For this review, take the finished solid that the model builds, in its own axes (mm). Face numbers are marked on the shaded views. Give positions to 0.01 mm unless a question says otherwise; leave off trailing zeros. Loops run counter-clockwise (first coordinate to the right, second up) from the corner with the lowest first, then second, coordinate; pieces in that order, holes last. Notation, with made-up numbers: (26, -25) - (74, -25) arc R16 ccw to (74, -14) - close; hole circle Ø8 at (-28.5, 68.5). An arc over 180 degrees is marked (long way). Answer in a Markdown table with one row per item.
```python
from build123d import *

# Parameters (mm, degrees)
ESQUISSE1_R        = 77.9
ESQUISSE1_R_2      = 2.25
ESQUISSE1_R_3      = 5
BOSS_EXTRU_1_DEPTH = 2


with BuildPart() as part:
    # Esquisse1 → Boss.-Extru.1 (new body)
    with BuildSketch(Plane.XY):
        with Locations((0.071120791, 0.517607885)):
            Circle(ESQUISSE1_R)
        with Locations((0.071120791, 73.017607885)):
            Circle(ESQUISSE1_R_2, mode=Mode.SUBTRACT)
        with Locations((72.571120791, 0.517607885)):
            Circle(ESQUISSE1_R_2, mode=Mode.SUBTRACT)
        with Locations((0.071120791, -71.982392115)):
            Circle(ESQUISSE1_R_2, mode=Mode.SUBTRACT)
        with Locations((-72.428879209, 0.517607885)):
            Circle(ESQUISSE1_R_2, mode=Mode.SUBTRACT)
        with Locations((0.071120791, 0.517607885)):
            Circle(ESQUISSE1_R_3, mode=Mode.SUBTRACT)
    extrude(amount=BOSS_EXTRU_1_DEPTH)


solid = part.part
```
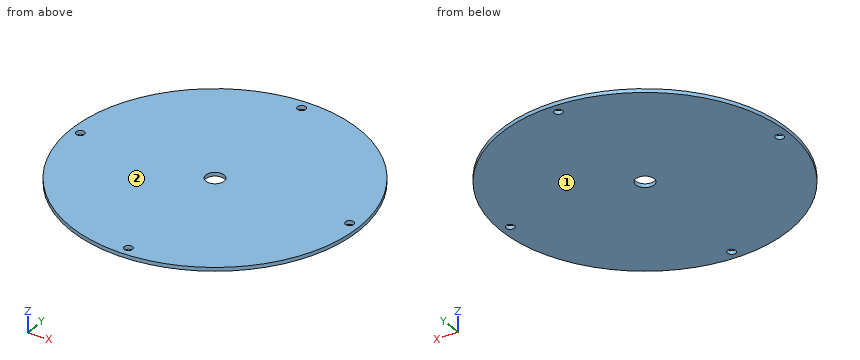
1. We need section A-A, the plane z = 1.3. Give the boundary of the cut face in (x, y).
Values:
| item | result |
|---|---|
| outline | circle Ø155.8 at (0.07, 0.52); hole circle Ø4.5 at (-72.43, 0.52); hole circle Ø10 at (0.07, 0.52); hole circle Ø4.5 at (0.07, -71.98); hole circle Ø4.5 at (0.07, 73.02); hole circle Ø4.5 at (72.57, 0.52) |
2. Mouldability with a two-part tool opening along Z and no side actions: class the marked faces 1 and 2 as released by +Z, released by -Z, zero draft, split by the parting line, or undercut.
Values:
| item | result |
|---|---|
| face 1 | released by -Z |
| face 2 | released by +Z |
3. We need section B-B, the plane x = -30. Give the boundary of the cut face in (y, z).
Values:
| item | result |
|---|---|
| outline | (-71.34, 0) - (72.38, 0) - (72.38, 2) - (-71.34, 2) - close |
4. We need section C-C, the plane y = -49. Give the boundary of the cut face in (x, z), and give its area (3 significant figures).
Values:
| item | result |
|---|---|
| outline | (-60.07, 0) - (60.21, 0) - (60.21, 2) - (-60.07, 2) - close |
| area | 241 mm^2 |
5. Wall thickness on line 1 (X direction, y = 4, z = 0.7); line 2 (X direction, y = 3, z = 0.3); line 3 (Y direction, x = 25, z = 0.35): over which ranges is each line inside the solid? List them lowest first. Write a range as [from, to].
Values:
| item | result |
|---|---|
| line 1 | x = [-77.75, -3.52], [3.66, 77.89] |
| line 2 | x = [-77.79, -4.27], [4.41, 77.93] |
| line 3 | y = [-73.29, 74.32] |
